from build123d import *

# Parameters (mm, degrees)
F0_W     = 1.4
F0_H     = 9.8
F1_DEPTH = 15.5
F2_DEPTH = 19.5
F3_DEPTH = 1
F4_DEPTH = 32.5


# Not quite as in the source:
# - ends of sketch curves that miss each other by under 0.0002 mm in the source are joined


with BuildPart() as f1:
    # F0 (on Top) → F1 (new body)
    with BuildSketch(Plane.XY):
        with BuildLine():
            Line((-32.0736061335, 18.2974073312), (-37.0736061335, 18.2974073312))
            Line((-37.0736061335, 18.2974073312), (-37.0736061335, 16.0974073312))
            Line((-37.0736061335, 16.0974073312), (-35.6736061335, 16.0974073312))
            Line((-35.6736061335, 16.0974073312), (-34.2736061335, 16.0974073312))
            Line((-34.2736061335, 16.0974073312), (-34.2736061335, 9.4129567733))
            ThreePointArc((-34.2736061335, 9.4129567733), (-34.2627799655, 9.2994922606), (-34.230692148, 9.1901223675))
            Line((-34.230692148, 9.1901223675), (-33.2244723711, 6.6745729254))
            ThreePointArc((-33.2244723711, 6.6745729254), (-33.0063342171, 6.402317089), (-32.6736057993, 6.2974395666))
            Line((-32.6736057993, 6.2974395666), (-32.6673863566, 6.2974073312))
            ThreePointArc((-32.6673863566, 6.2974073312), (-32.2471488287, 6.4753478956), (-32.0736061335, 6.8974073312))
            Line((-32.0736061335, 6.8974073312), (-32.0736061335, 18.2974073312))
        make_face()
        with Locations((-36.3736061335, 11.1974073312)):
            Rectangle(F0_W, F0_H)
        with BuildLine():
            Line((-35.6736061335, 6.2974073312), (-37.0736061335, 6.2974073312))
            Line((-37.0736061335, 6.2974073312), (-37.0736061335, 5.2974073312))
            Line((-37.0736061335, 5.2974073312), (-42.2844909944, 6.1658881413))
            ThreePointArc((-42.2844909944, 6.1658881413), (-42.8770439673, 6.0305679631), (-43.2034719774, 5.5178542706))
            ThreePointArc((-43.2034719774, 5.5178542706), (-43.1469979089, 5.0781395288), (-42.8650641349, 4.7360113048))
            ThreePointArc((-42.8650641349, 4.7360113048), (-38.9420533833, 0.8088724995), (-36.7058590055, -4.271665588))
            ThreePointArc((-36.7058590055, -4.271665588), (-36.5388782387, -4.5797772785), (-36.2106530565, -4.7025926688))
            Line((-36.2106530565, -4.7025926688), (-36.1736061335, -4.7025926688))
            ThreePointArc((-36.1736061335, -4.7025926688), (-35.8200527429, -4.5561460594), (-35.6736061335, -4.2025926688))
            Line((-35.6736061335, -4.2025926688), (-35.6736061335, 6.2974073312))
        make_face()
    extrude(amount=-F1_DEPTH)

    # F0 (on Top) → F2 (join)
    with BuildSketch(Plane.XY):
        with Locations((-36.3736061335, 11.1974073312)):
            Rectangle(F0_W, F0_H)
    extrude(amount=-F2_DEPTH)

    # F0 (on Top) → F3 (cut)
    with BuildSketch(Plane.XY):
        with Locations((-36.3736061335, 11.1974073312)):
            Rectangle(F0_W, F0_H)
        with BuildLine():
            Line((-35.6736061335, 6.2974073312), (-37.0736061335, 6.2974073312))
            Line((-37.0736061335, 6.2974073312), (-37.0736061335, 5.2974073312))
            Line((-37.0736061335, 5.2974073312), (-42.2844909944, 6.1658881413))
            ThreePointArc((-42.2844909944, 6.1658881413), (-42.8770439673, 6.0305679631), (-43.2034719774, 5.5178542706))
            ThreePointArc((-43.2034719774, 5.5178542706), (-43.1469979089, 5.0781395288), (-42.8650641349, 4.7360113048))
            ThreePointArc((-42.8650641349, 4.7360113048), (-38.9420533833, 0.8088724995), (-36.7058590055, -4.271665588))
            ThreePointArc((-36.7058590055, -4.271665588), (-36.5388782387, -4.5797772785), (-36.2106530565, -4.7025926688))
            Line((-36.2106530565, -4.7025926688), (-36.1736061335, -4.7025926688))
            ThreePointArc((-36.1736061335, -4.7025926688), (-35.8200527429, -4.5561460594), (-35.6736061335, -4.2025926688))
            Line((-35.6736061335, -4.2025926688), (-35.6736061335, 6.2974073312))
        make_face()
    extrude(amount=-F3_DEPTH, mode=Mode.SUBTRACT)

    # F0 (on Top) → F4 (join)
    with BuildSketch(Plane.XY):
        with BuildLine():
            Line((-32.0736061335, 18.2974073312), (-37.0736061335, 18.2974073312))
            Line((-37.0736061335, 18.2974073312), (-37.0736061335, 16.0974073312))
            Line((-37.0736061335, 16.0974073312), (-35.6736061335, 16.0974073312))
            Line((-35.6736061335, 16.0974073312), (-34.2736061335, 16.0974073312))
            Line((-34.2736061335, 16.0974073312), (-34.2736061335, 9.4129567733))
            ThreePointArc((-34.2736061335, 9.4129567733), (-34.2627799655, 9.2994922606), (-34.230692148, 9.1901223675))
            Line((-34.230692148, 9.1901223675), (-33.2244723711, 6.6745729254))
            ThreePointArc((-33.2244723711, 6.6745729254), (-33.0063342171, 6.402317089), (-32.6736057993, 6.2974395666))
            Line((-32.6736057993, 6.2974395666), (-32.6673863566, 6.2974073312))
            ThreePointArc((-32.6673863566, 6.2974073312), (-32.2471488287, 6.4753478956), (-32.0736061335, 6.8974073312))
            Line((-32.0736061335, 6.8974073312), (-32.0736061335, 18.2974073312))
        make_face()
    extrude(amount=-F4_DEPTH)


solid = f1.part
Check sheet for the modelled part. Datum: model origin and axes. Units: mm. A direction names the side the tool comes from. Round coordinates to 2 decimals unless told otherwise and drop trailing zeros. Order: outer loops, then holes, each group sorted by start corner. A loop starts at its lowest first (then second) coordinate and runs counter-clockwise, first axis right, second up.
(1) Scan lines: probe 1 along X at (y, z) = (14.25, -6); probe 2 along X at (y, z) = (10, -25.5); probe 3 along Z at (x, y) = (-39.5, 2.25). Record each from-to range of solid material in increasing order.
(2) Cross-section at C-C, the plane y = 8.5. Enter the section's corners in (x, z).
(3) Draft check along X on faces 1 (the flat face through (-38, 5, -1)), 2 (the cylindrical face through (-38.986, 0.873, -8.148)), 3 (the flat face through (-35.674, 6, -10)). Enter one of: pulls with the +X half, pulls with the -X half, needs draft (parallel to the pull), parting line crosses it, or undercut.
(4) Go/stop test with flat-tipped pins: P1, Ø6, axis at x = -38.5, z = -28, coming from the -Y side; P2, Ø4, axis at y = 13, z = -9, coming from the -X side; P3, Ø5, axis at x = -34.5, z = -20.5, coming from the -Y side. Record where each tip stops, or that it passes through.
(5) Cross-section at D-D, the plane x = -35. Enter the section's corners in (y, z).
(6) Access from +Z, -Z, +X, -X, +Y, -Y to the whole of each face (thin tool, end or side, straight path). Record for faces 4 (the flat face through (-33.735, 7.95, -16.022)), 5 (the flat face through (-38, 2, -15.5)), 6 (the flat face through (-36, 11, -19.5)).
(7) Cross-section at A-A, the plane y = 12. Enter the section's corners in (x, z), and give its area (3 significant figures).
Check sheet entries:
1. probe 1: x = -37.07 to -35.67, -34.27 to -32.07
1. probe 2: x = -34.27 to -32.07
1. probe 3: z = -15.5 to -1
2. outline: (-37.07, -19.5) - (-35.67, -19.5) - (-35.67, -1) - (-37.07, -1) - close; (-33.95, -32.5) - (-32.07, -32.5) - (-32.07, 0) - (-33.95, 0) - close
3. face 1: needs draft
3. face 2: pulls with the -X half
3. face 3: undercut
4. P1: stops at y = 16.1
4. P2: stops at x = -37.07
4. P3: stops at y = 6.3
5. outline: (16.1, -32.5) - (18.3, -32.5) - (18.3, 0) - (16.1, 0) - close
6. face 4: +Z, -Z, -Y
6. face 5: -Z, +X, -X, -Y
6. face 6: -Z, -X, -Y
7. outline: (-37.07, -19.5) - (-35.67, -19.5) - (-35.67, -1) - (-37.07, -1) - close; (-34.27, -32.5) - (-32.07, -32.5) - (-32.07, 0) - (-34.27, 0) - close
7. area: 97.4 mm2
